```python
from build123d import *

# Parameters (mm, degrees)
F0_W     = 46.4019156061
F0_H     = 38.3702367544
F1_DEPTH = 14.478
F2_R     = 5.08
F3_T     = -2.54
F4_R     = 5.5182295765
F5_DEPTH = 38.862


with BuildPart() as f1:
    # F0 (on Front) → F1 (new body, symmetric)
    with BuildSketch(Plane.XZ):
        with Locations((25.8178424556, 19.1851183772)):
            Rectangle(F0_W, F0_H)
    extrude(amount=F1_DEPTH, both=True)

    # F2
    f2_edges = [f1.edges().sort_by_distance(p)[0] for p in [
        (49.0188, 14.478, 19.185118),
        (49.0188, 0, 0),
        (2.616885, 0, 0),
        (25.817842, 14.478, 0),
        (2.616885, 14.478, 19.185118),
        (25.817842, 14.478, 38.370237),
        (49.0188, 0, 38.370237),
    ]]
    fillet(f2_edges, radius=F2_R)

    # F3
    f3_openings = [f1.faces().sort_by_distance(p)[0] for p in [
        (25.748559, -14.478, 19.241793),
    ]]
    offset(amount=F3_T, openings=f3_openings)

    # F4 (on face) → F5 (cut)
    with BuildSketch(Plane(origin=(0, 0, 0), x_dir=(1, 0, 0), z_dir=(0, 0, -1))):
        with Locations((22.9106154293, 3.8371770643)):
            Circle(F4_R)
    extrude(amount=-F5_DEPTH, mode=Mode.SUBTRACT)


solid = f1.part
```
Design review of the part built by this model. Coordinates are the model's own, in mm. A direction names the side the tool comes from. Coordinates: 2 decimals unless noted, no trailing zeros. Order: outer loops, then holes, each group sorted by start corner. A loop starts at its lowest first (then second) coordinate and runs counter-clockwise, first axis right, second up. Notation, with made-up numbers: M 79,2 L 106,2 A35 cw 106,41 Z; hole C 6.25,30.25 d4. An arc over 180 degrees is marked long. Answer as a JSON object with one key per item and string values. Group by question number.
1) Wall thickness on L1, parallel to Z at x = 8.5, y = -5; L2, parallel to X at y = 8.25, z = 15.5; L3, parallel to Y at x = 27, z = 32: over which ranges is each line inside the solid? List them lowest first.
2) Add section A-A, the plane y = -11.5. Write out the cut boundary in (x, z).
3) For pin 1 (14 mm diameter, centred on x = 17.5, z = 26, fed in from -Y); pin 2 (10 mm diameter, centred on x = 22.91, y = -3.84, fed in from -Z), all flat-tipped, find the tip position at first contact; note any pin that passes through.
4) Add section B-B, the plane y = 0.75. Write out the cut boundary in (x, z), then the cut area to 3 significant figures.
5) Mouldability with a two-part tool opening along Z and no side actions: class faces 3 (the cylindrical face through (47.57, 12.95, 19.38)), 4 (the cylindrical face through (4.066, -2.707, 1.528)), 5 (the cylindrical face through (5.881, -2.707, 3.304)), 6 (the flat face through (5.157, -3, 20)) as pulls with the +Z half, pulls with the -Z half, needs draft (parallel to the pull), parting line crosses it, or undercut.
6) Tool access review of faces 1 (the flat face through (46.479, -3, 19)), 2 (the flat face through (23, 3, 38.37)): name each direction out of +Z, -Z, +X, -X, +Y, -Y from which nothing blocks a thin tool from reaching the whole face with its end or side.
7) Add section C-C, the plane x = 16. Write out the cut boundary in (y, z).
8) Add section D-D, the plane z = 22.5. Write out the cut boundary in (x, y), then the cut area to 3 significant figures.
Computed values:
{
 "1": {"L1": "z = 0 to 2.54, 35.83 to 38.37", "L2": "x = 2.62 to 5.16, 46.48 to 49.02", "L3": "y = 11.94 to 14.48"},
 "2": {"outline": "M 2.62,5.08 A5.08 ccw 7.7,0 L 43.94,0 A5.08 ccw 49.02,5.08 L 49.02,33.29 A5.08 ccw 43.94,38.37 L 2.62,38.37 Z; hole M 5.16,5.08 A2.54 ccw 7.7,2.54 L 43.94,2.54 A2.54 ccw 46.48,5.08 L 46.48,33.29 A2.54 ccw 43.94,35.83 L 5.16,35.83 Z"},
 "3": {"pin 1": "stops at y = 11.94", "pin 2": "passes through"},
 "4": {"outline": "M 2.62,5.08 A5.08 ccw 7.7,0 L 19.84,0 L 19.84,2.54 L 7.7,2.54 A2.54 cw 5.16,5.08 L 5.16,35.83 L 19.84,35.83 L 19.84,38.37 L 2.62,38.37 Z; M 25.98,0 L 43.94,0 A5.08 ccw 49.02,5.08 L 49.02,33.29 A5.08 ccw 43.94,38.37 L 25.98,38.37 L 25.98,35.83 L 43.94,35.83 A2.54 cw 46.48,33.29 L 46.48,5.08 A2.54 cw 43.94,2.54 L 25.98,2.54 Z", "area": "361 mm^2"},
 "5": {"face 3": "needs draft", "face 4": "pulls with the -Z half", "face 5": "undercut", "face 6": "undercut"},
 "6": {"face 1": "-Y", "face 2": "+Z, +X, -X, +Y, -Y"},
 "7": {"outline": "M -14.48,0 L 9.4,0 A5.08 ccw 14.48,5.08 L 14.48,33.29 A5.08 ccw 9.4,38.37 L -14.48,38.37 L -14.48,35.83 L 9.4,35.83 A2.54 cw 11.94,33.29 L 11.94,5.08 A2.54 cw 9.4,2.54 L -14.48,2.54 Z"},
 "8": {"outline": "M 2.62,-14.48 L 5.16,-14.48 L 5.16,9.4 A2.54 cw 7.7,11.94 L 43.94,11.94 A2.54 cw 46.48,9.4 L 46.48,-14.48 L 49.02,-14.48 L 49.02,9.4 A5.08 ccw 43.94,14.48 L 7.7,14.48 A5.08 ccw 2.62,9.4 Z", "area": "244 mm^2"}
}
